Work out the finished part from the listing and answer in its coordinate system (mm). A direction names the side the tool comes from. Give positions to 0.01 mm unless a question says otherwise; leave off trailing zeros. Loops run counter-clockwise (first coordinate to the right, second up) from the corner with the lowest first, then second, coordinate; pieces in that order, holes last. Notation, with made-up numbers: (86.25, -5.75) -> (127.25, -5.75) arc R8 ccw to (127.25, 2.25) -> close; hole circle Ø11 at (-19.5, 71.25). An arc over 180 degrees is marked (long way). Answer as CSV lines item,"result". Start each with the question number.
1. Flat-ended cylindrical pins translate along their axes: pin 1 Ø5 at (y, z) = (-3, 16) entering from +X (3 decimals); pin 2 Ø2 at (x, y) = (-0.5, -1) entering from -Z; pin 3 Ø2.5 at (x, z) = (-0.5, 15) entering from -Y. Find the tip coordinate at first contact, or state that the pin passes through.
2. Find section A-A, the plane y = 3.25. Give the vertices of the cut face in (x, z) (1 decimal), and give its area (3 significant figures).
3. Determine the mould class of faces 6 (the face through (0, -3.81, 6)), 7 (the face through (-0.07, 3.92, 4.38)), 8 (the face through (0, 0, 7.112)) for opening direction Z: +Z half, -Z half, draft (parallel to the pull), parting line (faces both ways), or undercut.
4. A tool of negligible diameter and unlimited length cuts with its end or side. For faces 1 (the face through (0, 1.651, 14)), 2 (the face through (0, -4, 8.382)), 3 (the face through (-1.905, 0, 14)), 4 (the face through (4.445, -2, 4)), 5 (the face through (0, -1.651, 14)), from which of +Z, -Z, +X, -X, +Y, -Y can it reach the whole face along a straight path? Write none if from no direction.
5. Find section C-C, the plane z = 3.75. Give the vertices of the cut face in (x, y) (3 decimals).
6. Find the intervals of material crossed by line 1 along X through (y, z) = (-2, 5.5) (3 decimals); line 2 along X through (y, z) = (2.5, 5.25); line 3 along Y through (x, z) = (-0.5, 16.5), in increasing order.
7. Find section D-D, the plane z = 16. Give the vertices of the cut face in (x, y) (3 decimals).
from build123d import *

# Parameters (mm, degrees)
SKETCH1_W               = 10.16
SKETCH1_H               = 9.652
BOSS_EXTRUDE1_DEPTH     = 7.112
CUT_EXTRUDE1_DEPTH      = 14.021061708
CUT_EXTRUDE1_DEPTH_BACK = 14.021061708
SKETCH2_R               = 1.5875
SKETCH7_W               = 10.16
SKETCH7_H               = 9.652
BOSS_EXTRUDE3_DEPTH     = 1.27
FILLET1_R               = 0.635
FILLET3_R               = 0.635
FILLET4_R               = 0.381
CUT_EXTRUDE3_DEPTH      = 14.574749537
CUT_EXTRUDE3_DEPTH_BACK = 14.574749537
FILLET9_R               = 0.254
CUT_EXTRUDE7_DEPTH      = 9.654656319
SKETCH14_W              = 3.81
SKETCH14_H              = 3.302
BOSS_EXTRUDE4_DEPTH     = 10.16
FILLET14_R              = 1.27
FILLET15_R              = 0.254


# Some blends are built 0.0001 mm under size
with BuildPart() as part:
    # Sketch1 → Boss-Extrude1 (new body)
    with BuildSketch(Plane.XY):
        Rectangle(SKETCH1_W, SKETCH1_H)
        Polygon((-4.445, -3.81), (4.445, -3.81), (4.445, -1.016), (3.429, -1.016), (3.429, 3.048), (-3.429, 3.048), (-3.429, -1.016), (-4.445, -1.016), align=None, mode=Mode.SUBTRACT)
    extrude(amount=BOSS_EXTRUDE1_DEPTH)

    # Sketch2 → Cut-Extrude1 (cut, two sides: drawn at the far end of the back side and taken through both)
    with BuildSketch(Plane(origin=(0, 4.826, 0), x_dir=(1, 0, 0), z_dir=(0, 1, 0)).offset(-CUT_EXTRUDE1_DEPTH_BACK)):
        with Locations(Location((0, -2.794, 0), (0, 0, 90))):
            Circle(SKETCH2_R)
    extrude(amount=CUT_EXTRUDE1_DEPTH + CUT_EXTRUDE1_DEPTH_BACK, mode=Mode.SUBTRACT)

    # Sketch7 → Boss-Extrude3 (add)
    with BuildSketch(Plane.XY.offset(7.112)):
        Rectangle(SKETCH7_W, SKETCH7_H)
    extrude(amount=BOSS_EXTRUDE3_DEPTH)

    # Fillet1
    fillet1_edges = [part.edges().sort_by_distance(p)[0] for p in [
        (-5.08, 0, 0),
        (0, 4.826, 0),
        (5.08, 0, 0),
    ]]
    fillet(fillet1_edges, radius=FILLET1_R - 0.0001)  # a hair under: the kernel refuses the full size

    # Fillet3
    # the kernel refuses this fillet: 0.635 mm, written as the material it takes off along each edge
    with BuildSketch(Plane(origin=(4.445, 4.191, 0), x_dir=(0, 1, 0), z_dir=(-1, 0, 0))) as fillet3_piece_1:
        with BuildLine():
            CenterArc((0.0001, -0.6349), 0.6349, 0, 90)
            Line((0.635, -0.6349), (0.635, 0))
            Line((0.635, 0), (0.0001, 0))
        make_face()
    revolve(axis=Axis((4.445, 4.191, 0), (0, 0, -1)), revolution_arc=90, mode=Mode.SUBTRACT)
    with BuildSketch(Plane(origin=(-4.445, 4.191, 0), x_dir=(-1, 0, 0), z_dir=(0, -1, 0))) as fillet3_piece_2:
        with BuildLine():
            CenterArc((0.0001, -0.6349), 0.6349, 0, 90)
            Line((0.635, -0.6349), (0.635, 0))
            Line((0.635, 0), (0.0001, 0))
        make_face()
    revolve(axis=Axis((-4.445, 4.191, 0), (0, 0, -1)), revolution_arc=90, mode=Mode.SUBTRACT)
    with BuildSketch(Plane(origin=(-4.445, -4.191, 7.747), x_dir=(0, 0, 1), z_dir=(-1, 0, 0))) as fillet3_piece_3_section:
        Polygon((0, 0), (FILLET3_R * 1.02, 0), (FILLET3_R * 1.02, -FILLET3_R * 1.02), (0, -FILLET3_R * 1.02), align=None)
    fillet3_piece_3 = extrude(amount=FILLET3_R * 1.02, mode=Mode.PRIVATE)
    fillet3_piece_3 = fillet3_piece_3 - Plane(origin=(-4.445, -4.191, 7.747), x_dir=(0, 0.7071067811865475, -0.7071067811865475), z_dir=(-1, 0, 0)) * Sphere(FILLET3_R, mode=Mode.PRIVATE)
    add(fillet3_piece_3, mode=Mode.SUBTRACT)
    with BuildSketch(Plane(origin=(-4.445, 4.191, 7.747), x_dir=(-1, 0, 0), z_dir=(0, 1, 0))) as fillet3_piece_4_section:
        Polygon((0, 0), (FILLET3_R * 1.02, 0), (FILLET3_R * 1.02, FILLET3_R * 1.02), (0, FILLET3_R * 1.02), align=None)
    fillet3_piece_4 = extrude(amount=FILLET3_R * 1.02, mode=Mode.PRIVATE)
    fillet3_piece_4 = fillet3_piece_4 - Plane(origin=(-4.445, 4.191, 7.747), x_dir=(0.7071067811865475, 0, -0.7071067811865475), z_dir=(0, 1, 0)) * Sphere(FILLET3_R, mode=Mode.PRIVATE)
    add(fillet3_piece_4, mode=Mode.SUBTRACT)
    with BuildSketch(Plane(origin=(4.445, -4.191, 7.747), x_dir=(1, 0, 0), z_dir=(0, 0, 1))) as fillet3_piece_5_section:
        Polygon((0, 0), (FILLET3_R * 1.02, 0), (FILLET3_R * 1.02, -FILLET3_R * 1.02), (0, -FILLET3_R * 1.02), align=None)
    fillet3_piece_5 = extrude(amount=FILLET3_R * 1.02, mode=Mode.PRIVATE)
    fillet3_piece_5 = fillet3_piece_5 - Plane(origin=(4.445, -4.191, 7.747), x_dir=(-0.7071067811865476, 0.7071067811865475, 0), z_dir=(0, 0, 1)) * Sphere(FILLET3_R, mode=Mode.PRIVATE)
    add(fillet3_piece_5, mode=Mode.SUBTRACT)
    with BuildSketch(Plane(origin=(4.445, 4.191, 7.747), x_dir=(0, 0, 1), z_dir=(0, 1, 0))) as fillet3_piece_6_section:
        Polygon((0, 0), (FILLET3_R * 1.02, 0), (FILLET3_R * 1.02, FILLET3_R * 1.02), (0, FILLET3_R * 1.02), align=None)
    fillet3_piece_6 = extrude(amount=FILLET3_R * 1.02, mode=Mode.PRIVATE)
    fillet3_piece_6 = fillet3_piece_6 - Plane(origin=(4.445, 4.191, 7.747), x_dir=(-0.7071067811865475, 0, -0.7071067811865475), z_dir=(0, 1, 0)) * Sphere(FILLET3_R, mode=Mode.PRIVATE)
    add(fillet3_piece_6, mode=Mode.SUBTRACT)
    with BuildSketch(Plane(origin=(-5.08, -4.191, 8.382), x_dir=(0, 0, -1), z_dir=(0, 1, 0))) as fillet3_piece_7:
        with BuildLine():
            CenterArc((FILLET3_R, -FILLET3_R), FILLET3_R, 90, 90)
            Line((0, -FILLET3_R), (-FILLET3_R * 0.02, -FILLET3_R))
            Line((-FILLET3_R * 0.02, -FILLET3_R), (-FILLET3_R * 0.02, FILLET3_R * 0.02))
            Line((-FILLET3_R * 0.02, FILLET3_R * 0.02), (FILLET3_R, FILLET3_R * 0.02))
            Line((FILLET3_R, FILLET3_R * 0.02), (FILLET3_R, 0))
        make_face()
    extrude(amount=8.382, mode=Mode.SUBTRACT)
    with BuildSketch(Plane(origin=(4.445, -4.826, 8.382), x_dir=(0, 1, 0), z_dir=(-1, 0, 0))) as fillet3_piece_8:
        with BuildLine():
            CenterArc((FILLET3_R, FILLET3_R), FILLET3_R, 180, 90)
            Line((0, FILLET3_R), (-FILLET3_R * 0.02, FILLET3_R))
            Line((-FILLET3_R * 0.02, FILLET3_R), (-FILLET3_R * 0.02, -FILLET3_R * 0.02))
            Line((-FILLET3_R * 0.02, -FILLET3_R * 0.02), (FILLET3_R, -FILLET3_R * 0.02))
            Line((FILLET3_R, -FILLET3_R * 0.02), (FILLET3_R, 0))
        make_face()
    extrude(amount=8.89, mode=Mode.SUBTRACT)
    with BuildSketch(Plane(origin=(5.08, 4.191, 8.382), x_dir=(-1, 0, 0), z_dir=(0, -1, 0))) as fillet3_piece_9:
        with BuildLine():
            CenterArc((FILLET3_R, FILLET3_R), FILLET3_R, 180, 90)
            Line((0, FILLET3_R), (-FILLET3_R * 0.02, FILLET3_R))
            Line((-FILLET3_R * 0.02, FILLET3_R), (-FILLET3_R * 0.02, -FILLET3_R * 0.02))
            Line((-FILLET3_R * 0.02, -FILLET3_R * 0.02), (FILLET3_R, -FILLET3_R * 0.02))
            Line((FILLET3_R, -FILLET3_R * 0.02), (FILLET3_R, 0))
        make_face()
    extrude(amount=8.382, mode=Mode.SUBTRACT)
    with BuildSketch(Plane(origin=(-4.445, 4.826, 8.382), x_dir=(0, 0, -1), z_dir=(1, 0, 0))) as fillet3_piece_10:
        with BuildLine():
            CenterArc((FILLET3_R, -FILLET3_R), FILLET3_R, 90, 90)
            Line((0, -FILLET3_R), (-FILLET3_R * 0.02, -FILLET3_R))
            Line((-FILLET3_R * 0.02, -FILLET3_R), (-FILLET3_R * 0.02, FILLET3_R * 0.02))
            Line((-FILLET3_R * 0.02, FILLET3_R * 0.02), (FILLET3_R, FILLET3_R * 0.02))
            Line((FILLET3_R, FILLET3_R * 0.02), (FILLET3_R, 0))
        make_face()
    extrude(amount=8.89, mode=Mode.SUBTRACT)
    with BuildSketch(Plane(origin=(6.0326, -4.826, 0), x_dir=(0, 0, 1), z_dir=(-1, 0, 0))) as fillet3_piece_11:
        with BuildLine():
            CenterArc((FILLET3_R, FILLET3_R), FILLET3_R, 180, 90)
            Line((0, FILLET3_R), (-FILLET3_R * 0.02, FILLET3_R))
            Line((-FILLET3_R * 0.02, FILLET3_R), (-FILLET3_R * 0.02, -FILLET3_R * 0.02))
            Line((-FILLET3_R * 0.02, -FILLET3_R * 0.02), (FILLET3_R, -FILLET3_R * 0.02))
            Line((FILLET3_R, -FILLET3_R * 0.02), (FILLET3_R, 0))
        make_face()
    extrude(amount=12.0652, mode=Mode.SUBTRACT)
    with BuildSketch(Plane(origin=(4.4451, -4.826, 0.6349), x_dir=(0, 0, -1), z_dir=(-1, 0, 0))) as fillet3_piece_12:
        with BuildLine():
            CenterArc((-0.0001, -0.635), FILLET3_R, 0, 89.990977043)
            Line((0.6349, -0.635), (0.6476, -0.635))
            Line((0.6476, -0.635), (0.6476, 0.0127))
            Line((0.6476, 0.0127), (0, 0.0127))
            Line((0, 0.0127), (0, -8e-09))
        make_face()
    revolve(axis=Axis((4.4451, -4.826, 0.6349), (0, -1, 0)), revolution_arc=90, mode=Mode.SUBTRACT)
    with BuildSketch(Plane(origin=(-4.4451, -4.826, 0.6349), x_dir=(0, 0, -1), z_dir=(1, 0, 0))) as fillet3_piece_13:
        with BuildLine():
            CenterArc((-0.0001, 0.635), FILLET3_R, 270.009022957, 89.990977043)
            Line((0.6349, 0.635), (0.6476, 0.635))
            Line((0.6476, 0.635), (0.6476, -0.0127))
            Line((0.6476, -0.0127), (0, -0.0127))
            Line((0, -0.0127), (0, 8e-09))
        make_face()
    revolve(axis=Axis((-4.4451, -4.826, 0.6349), (0, 1, 0)), revolution_arc=90, mode=Mode.SUBTRACT)
    with BuildSketch(Plane(origin=(5.08, -4.826, 7.747), x_dir=(0, 1, 0), z_dir=(0, 0, -1)), Plane(origin=(-5.08, -4.826, -0.9526), x_dir=(0, 1, 0), z_dir=(0, 0, 1))) as fillet3_piece_14:
        with BuildLine():
            CenterArc((FILLET3_R, -FILLET3_R), FILLET3_R, 90, 90)
            Line((0, -FILLET3_R), (-FILLET3_R * 0.02, -FILLET3_R))
            Line((-FILLET3_R * 0.02, -FILLET3_R), (-FILLET3_R * 0.02, FILLET3_R * 0.02))
            Line((-FILLET3_R * 0.02, FILLET3_R * 0.02), (FILLET3_R, FILLET3_R * 0.02))
            Line((FILLET3_R, FILLET3_R * 0.02), (FILLET3_R, 0))
        make_face()
    extrude(amount=8.6996, mode=Mode.SUBTRACT)
    with BuildSketch(Plane(origin=(-5.08, 4.826, 0), x_dir=(1, 0, 0), z_dir=(0, 0, 1)), Plane(origin=(5.08, 4.826, 7.747), x_dir=(-1, 0, 0), z_dir=(0, 0, -1))) as fillet3_piece_15:
        with BuildLine():
            CenterArc((FILLET3_R, -FILLET3_R), FILLET3_R, 90, 90)
            Line((0, -FILLET3_R), (-FILLET3_R * 0.02, -FILLET3_R))
            Line((-FILLET3_R * 0.02, -FILLET3_R), (-FILLET3_R * 0.02, FILLET3_R * 0.02))
            Line((-FILLET3_R * 0.02, FILLET3_R * 0.02), (FILLET3_R, FILLET3_R * 0.02))
            Line((FILLET3_R, FILLET3_R * 0.02), (FILLET3_R, 0))
        make_face()
    extrude(amount=7.747, mode=Mode.SUBTRACT)

    # Fillet4
    fillet4_edges = [part.edges().sort_by_distance(p)[0] for p in [
        (3.429, -1.016, 3.556),
        (-3.429, -1.016, 3.556),
    ]]
    fillet(fillet4_edges, radius=FILLET4_R)

    # Sketch11 → Cut-Extrude3 (cut, two sides: drawn at the far end of the back side and taken through both)
    with BuildSketch(Plane.ZY.offset(-4.445).offset(-CUT_EXTRUDE3_DEPTH_BACK)):
        Polygon((0, -3.81), (5.08, -3.81), (5.08, -4.064), (10.16, -4.826), (0, -4.826), align=None)
    extrude(amount=CUT_EXTRUDE3_DEPTH + CUT_EXTRUDE3_DEPTH_BACK, mode=Mode.SUBTRACT)

    # Fillet9
    fillet9_edges = [part.edges().sort_by_distance(p)[0] for p in [
        (-4.445, -3.81, 6.096),
        (4.445, -3.81, 6.096),
        (0, -3.81, 7.112),
    ]]
    fillet(fillet9_edges, radius=FILLET9_R)

    # Sketch13 → Cut-Extrude7 (cut, through all)
    with BuildSketch(Plane(origin=(0, 0, 5.08), x_dir=(-1, 0, 0), z_dir=(0, 0, -1))):
        Polygon((-5.08, -3.81), (-5.08, -4.826), (-2.54, -4.826), align=None)
        Polygon((5.08, -3.81), (5.08, -4.826), (2.032, -4.826), align=None)
    extrude(amount=-CUT_EXTRUDE7_DEPTH, mode=Mode.SUBTRACT)

    # Sketch14 → Boss-Extrude4 (add)
    with BuildSketch(Plane.XY.offset(8.382)):
        Rectangle(SKETCH14_W, SKETCH14_H)
    extrude(amount=BOSS_EXTRUDE4_DEPTH)

    # Fillet14
    fillet14_edges = [part.edges().sort_by_distance(p)[0] for p in [
        (0, 1.651, 8.382),
        (-1.905, 0, 8.382),
        (0, -1.651, 8.382),
        (1.905, 0, 8.382),
    ]]
    fillet(fillet14_edges, radius=FILLET14_R)

    # Fillet15
    fillet15_edges = [part.edges().sort_by_distance(p)[0] for p in [
        (1.905, 1.651, 14.097),
        (-1.905, 1.651, 14.097),
        (-1.905, -1.651, 14.097),
        (1.905, -1.651, 14.097),
        (0, 1.651, 18.542),
        (-1.905, 0, 18.542),
        (0, -1.651, 18.542),
        (1.905, 0, 18.542),
        (2.354517888, 2.100517888, 8.682614059),
        (2.354517888, -2.100517888, 8.682614059),
        (-2.354517888, 2.100517888, 8.682614059),
        (-2.354517888, -2.100517888, 8.682614059),
    ]]
    fillet(fillet15_edges, radius=FILLET15_R)


solid = part.part
Resolved:
1,pin 1,"stops at x = 1.905"
1,pin 2,"stops at z = 7.11"
1,pin 3,"stops at y = -1.65"
2,outline,"(-5.1, 0.6) arc R0.6 ccw to (-4.4, 0) -> (4.4, 0) arc R0.6 ccw to (5.1, 0.6) -> (5.1, 7.7) arc R0.6 ccw to (4.4, 8.4) -> (-4.4, 8.4) arc R0.6 ccw to (-5.1, 7.7) -> close; hole circle Ø3.2 at (0, 2.8)"
2,area,"76.9 mm^2"
3,face 6,"draft"
3,face 7,"undercut"
3,face 8,"-Z half"
4,face 1,"+Z, +X, -X, +Y"
4,face 2,"+Z"
4,face 3,"+Z, -X, +Y, -Y"
4,face 4,"-Z"
4,face 5,"+Z, +X, -X, -Y"
5,outline,"(-5.08, -3.81) -> (-4.445, -3.81) -> (-4.445, -1.016) -> (-3.81, -1.016) arc R0.381 ccw to (-3.429, -0.635) -> (-3.429, 3.048) -> (-1.267, 3.048) -> (-1.267, 4.826) -> (-4.445, 4.826) arc R0.635 ccw to (-5.08, 4.191) -> close; (1.267, 3.048) -> (3.429, 3.048) -> (3.429, -0.635) arc R0.381 ccw to (3.81, -1.016) -> (4.445, -1.016) -> (4.445, -3.81) -> (5.08, -3.81) -> (5.08, 4.191) arc R0.635 ccw to (4.445, 4.826) -> (1.267, 4.826) -> close"
6,line 1,"x = -5.08 to -4.445, 4.445 to 5.08"
6,line 2,"x = -5.08 to -3.43, 3.43 to 5.08"
6,line 3,"y = -1.65 to 1.65"
7,outline,"(-1.905, -1.397) arc R0.254 ccw to (-1.651, -1.651) -> (1.651, -1.651) arc R0.254 ccw to (1.905, -1.397) -> (1.905, 1.397) arc R0.254 ccw to (1.651, 1.651) -> (-1.651, 1.651) arc R0.254 ccw to (-1.905, 1.397) -> close"
